Read the model definition and answer for the solid it produces. Units are mm, in the model's axes. Coordinates: 2 decimals unless noted, no trailing zeros. Loops run counter-clockwise (first coordinate to the right, second up) from the corner with the lowest first, then second, coordinate; pieces in that order, holes last. Notation, with made-up numbers: (73.5, 17.25) - (92.5, 17.25) arc R20 cw to (92.5, 29.25) - close; hole circle Ø11 at (-5, -21). An arc over 180 degrees is marked (long way). One line per item, written item: value. Start each with the question number.
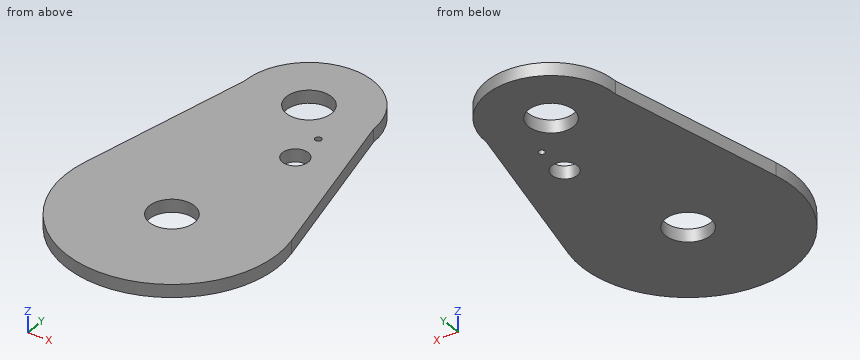
Autodesk Inventor part; units mm, degrees
ref_plane "YZ Plane" through (0, 0, 0) normal (1, 0, 0) x (0, 1, 0)
ref_plane "XZ Plane" through (0, 0, 0) normal (0, 1, 0) x (-1, 0, 0)
ref_plane "XY Plane" through (0, 0, 0) normal (0, 0, 1) x (1, 0, 0)
sketch "Sketch1" plane through (0, 0, 0) normal (0, 0, 1) x (1, 0, 0)
  arc A0 (-32.2108, 7.1739) -> (32.2108, 7.1739) centre (0, 0) ccw
  arc A1 (20, 62) -> (-20, 62) centre (0, 62) ccw
  line L0 (20, 62) -> (32.2108, 7.1739)
  line L1 (-20, 62) -> (-32.2108, 7.1739)
  circle A2 centre (0, 0) radius 7
  circle A3 centre (0, 62) radius 7
  circle A4 centre (11, 39.7881) radius 4
  circle A5 centre (11, 50.1761) radius 1
  dimension "d0" = 66
  dimension "d1" = 40
  dimension "d2" = 62
  dimension "d3" = 14
  dimension "d4" = 14
  dimension "d5" = 8
  dimension "d6" = 2
  dimension "d7" = 11
extrude "Extrusion1" add sketch "Sketch1" along normal blind 4
properties part number "Placa de soporte"
1) Section B-B, the plane x = 0 is taken. Determine the outline of the cut face in (y, z), and give its area (3 significant figures).
2) Section A-A, the plane y = 0 is taken. Determine the outline of the cut face in (x, z), and give its area (3 significant figures).
3) Section D-D, the plane x = -14.5 is taken. Determine the outline of the cut face in (y, z), and give its area (3 significant figures).
4) Section C-C, the plane z = 0.7 is taken. Determine the outline of the cut face in (x, y).
5) Flat-ended cylindrical pins translate along their axes: P1, Ø8.5, axis at x = 0, y = 0, coming from the +Z side; P2, Ø1.5, axis at y = -2, z = 3.5, coming from the -X side; P3, Ø1, axis at x = 19.5, y = -19.5, coming from the -Z side. Find the tip coordinate at first contact, or state that the pin passes through.
6) Straight lines are drawn through the part: L1, parallel to Y at x = 11, z = 2.3; L2, parallel to X at y = 65, z = 3.3; L3, parallel to X at y = 63, z = 2. For each, find the intervals that lie inside material, in ascending order.
Answer below:
1. outline: (-33, 0) - (-7, 0) - (-7, 4) - (-33, 4) - close; (7, 0) - (55, 0) - (55, 4) - (7, 4) - close; (69, 0) - (82, 0) - (82, 4) - (69, 4) - close
1. area: 348 mm2
2. outline: (-33, 0) - (-7, 0) - (-7, 4) - (-33, 4) - close; (7, 0) - (33, 0) - (33, 4) - (7, 4) - close
2. area: 208 mm2
3. outline: (-29.64, 0) - (75.77, 0) - (75.77, 4) - (-29.64, 4) - close
3. area: 422 mm2
4. outline: (-32.21, 7.17) arc R33 ccw (long way) to (32.21, 7.17) - (20, 62) arc R20 ccw to (-20, 62) - close; hole circle Ø14 at (0, 0); hole circle Ø14 at (0, 62); hole circle Ø8 at (11, 39.79); hole circle Ø2 at (11, 50.18)
5. P1: through
5. P2: x = -32.98
5. P3: z = 0
6. L1: -31.11 to 35.79, 43.79 to 49.18, 51.18 to 78.7
6. L2: -19.77 to -6.32, 6.32 to 19.77
6. L3: -19.97 to -6.93, 6.93 to 19.97
